Check sheet for the drawn part. Datum: minimum x, y, z corner. Units: mm. Round coordinates to 2 decimals unless told otherwise and drop trailing zeros. Write each loop counter-clockwise with the first axis right and the second up, starting at its lowest first coordinate (ties: lowest second). Pieces come first, ordered by that corner, then holes. Notation, with made-up numbers: (15.25, 14) -> (38.25, 14) arc R10 cw to (38.25, 29) -> close; hole circle Ø8 at (-32, -11). An arc over 180 degrees is marked (long way). Use a Markdown table: item, result.
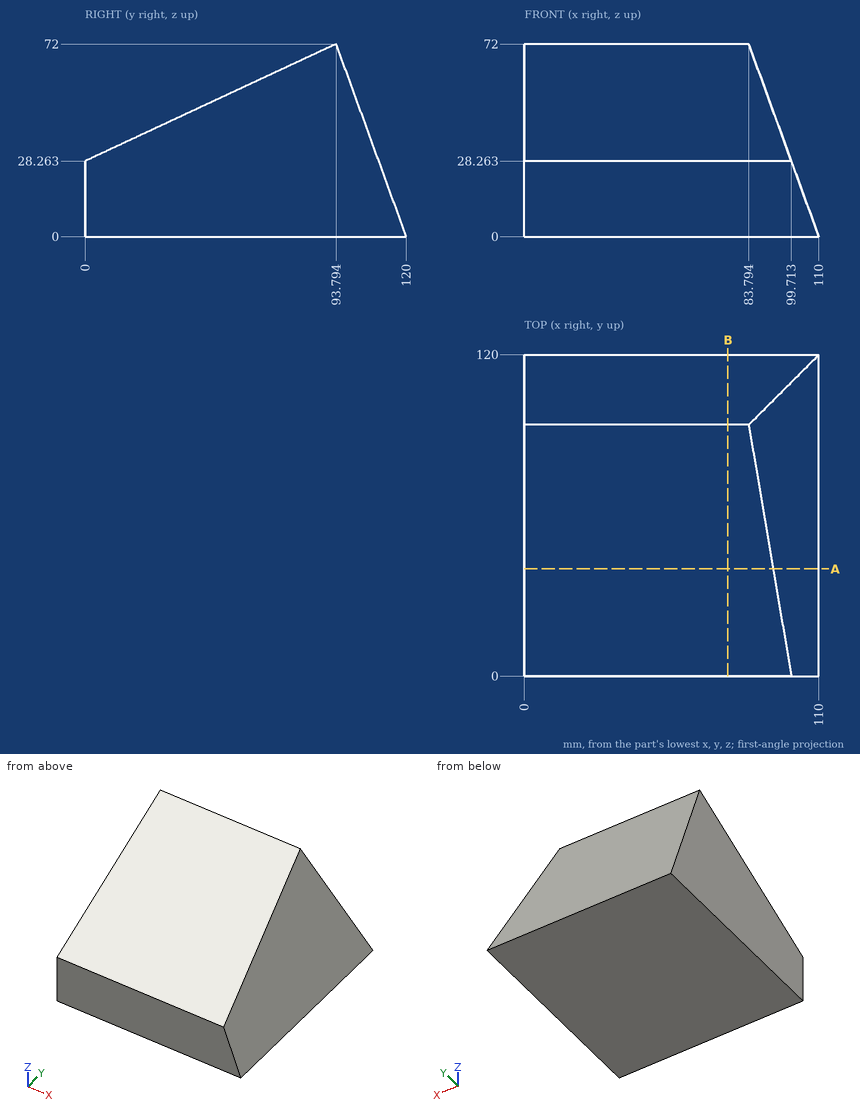
(1) Section check A-A on y = 40. Record the cut outline in (x, z).
A:
| item | result |
|---|---|
| outline | (0, 0) -> (110, 0) -> (92.92, 46.92) -> (0, 46.92) -> close |
(2) Section check B-B on x = 76. Record the cut outline in (y, z).
A:
| item | result |
|---|---|
| outline | (0, 0) -> (120, 0) -> (93.79, 72) -> (0, 28.26) -> close |
(3) Thickness scan on line 1 (Z direction, x = 61.5, y = 32) (1 decimal); line 2 (Y direction, x = 53.5, z = 47); line 3 (X direction, y = 62.5, z = 43.5). Record the ranges inside material, lowest first.
A:
| item | result |
|---|---|
| line 1 | z = 0 to 43.2 |
| line 2 | y = 40.18 to 102.89 |
| line 3 | x = 0 to 94.17 |
(4) Gauge pin test, flat ends, axial feed: pin 1 Ø3 at (x, z) = (93.5, 19) entering from +Y; pin 2 Ø12 at (x, z) = (72, 31.5) entering from +Y; pin 3 Ø3 at (y, z) = (41.5, 27.5) entering from +X. Record the tip position at first contact, or that the pin passes through.
A:
| item | result |
|---|---|
| pin 1 | stops at y = 113.63 |
| pin 2 | stops at y = 110.72 |
| pin 3 | stops at x = 100.54 |
